The model under review builds one solid part; all positions refer to its coordinate system, in mm. A direction names the side the tool comes from. Coordinates: 2 decimals unless noted, no trailing zeros. Order: outer loops, then holes, each group sorted by start corner. A loop starts at its lowest first (then second) coordinate and runs counter-clockwise, first axis right, second up. Notation, with made-up numbers: M 31.5,57 L 83.5,57 A20 ccw 83.5,89 Z; hole C -28.75,-34.75 d1. An arc over 180 degrees is marked long. One line per item, written item: value.
```python
from build123d import *

# Parameters (mm, degrees)
SKETCH_2_R     = 5
SKETCH_2_R_2   = 3
CHAMFER_1_SIZE = 1


with BuildPart() as part:
    # По траектории1: sweep along a path in Эскиз1
    with BuildLine(Plane.XY) as sweep_1_path:
        Line((0, 0), (105, 0))
        ThreePointArc((105, 0), (123.47759065, -12.346331353), (119.142135624, -34.142135624))
        Line((119.142135624, -34.142135624), (95.857864376, -57.426406871))
        ThreePointArc((95.857864376, -57.426406871), (91.52240935, -63.914873848), (90, -71.568542495))
        Line((90, -71.568542495), (90, -100))
    # Эскиз2 → По траектории1 (sweep)
    with BuildSketch(Plane(origin=(0, 0, 0), x_dir=(0, 0, -1), z_dir=(1, 0, 0))):
        Circle(SKETCH_2_R)
        Circle(SKETCH_2_R_2, mode=Mode.SUBTRACT)
    sweep(path=sweep_1_path.line)

    # Фаска1
    chamfer_1_edges = [part.edges().sort_by_distance(p)[0] for p in [
        (90, -100, 5),
        (0, 0, 5),
    ]]
    chamfer(chamfer_1_edges, length=CHAMFER_1_SIZE)


solid = part.part
```
(1) For L1, parallel to Y at x = 81, z = 0; L2, parallel to X at y = -85.25, z = 0; L3, parallel to Y at x = 101, z = 1, list the stretches that pass through material, from the lowest coordinate up.
Geometry results:
L1: y = -5 to -3, 3 to 5
L2: x = 85 to 87, 93 to 95
L3: y = -59.21 to -56.28, -48.28 to -45.36, -4.9 to -2.83, 2.83 to 4.9
(2) We need section D-D, the plane y = -78. State the section outline as (x, z) points.
Geometry results:
outline: C 90,0 d10; hole C 90,0 d6
(3) We need section C-C, the plane x = 8. State the section outline as (y, z) points.
Geometry results:
outline: C 0,0 d10; hole C 0,0 d6
(4) Mouldability with a two-part tool opening along Y and no side actions: class faces 1 (the flat face through (93, -100, -1)), 2 (the cylindrical face through (85.12, -85.48, 1.08)), 3 (the cylindrical face through (103.886, -42.496, 1.084)) as +Y half, -Y half, draft (parallel to the pull), parting line (faces both ways), or undercut.
Geometry results:
face 1: -Y half
face 2: draft
face 3: undercut
(5) Tool access review of faces 4 (the flat face through (0, -3, 1)), 5 (the cylindrical face through (87.07, -85.98, 0.65)), 6 (the cylindrical face through (53.73, -4.88, 1.08)): name each direction out of +Z, -Z, +X, -X, +Y, -Y from which nothing blocks a thin tool from reaching the whole face with its end or side.
Geometry results:
face 4: +Z, -Z, -X, +Y, -Y
face 5: -Y
face 6: -X
(6) We need section A-A, the plane x = 90. Count the separate pieces of the cut face and the enclosed holes in it, plus the area to 3 significant figures.
Geometry results:
separate pieces: 2
enclosed holes: 1
area: 234 mm2
(7) Insertion check: pin 1 Ø2 at (x, z) = (82.5, -3) entering from -Y; pin 2 Ø2 at (x, z) = (102, -1) entering from -Y; pin 3 Ø5 at (y, z) = (0, 0) entering from +X. Each pin has a flat end and moves straight along its axis. Give the tip position at first contact, or say it passes through.
Geometry results:
pin 1: stops at y = -4.58
pin 2: stops at y = -59.24
pin 3: stops at x = 122.85
(8) We need section B-B, the plane z = 0. State the section outline as (x, y) points, plus the area to 3 significant figures.
Geometry results:
outline: M 0,-4 L 1,-5 L 105,-5 A15 cw 115.61,-30.61 L 92.32,-53.89 A25 ccw 85,-71.57 L 85,-99 L 86,-100 L 87,-100 L 87,-71.57 A23 cw 93.74,-55.31 L 117.02,-32.02 A17 ccw 105,-3 L 0,-3 Z; M 0,3 L 105,3 A23 cw 121.26,-36.26 L 97.98,-59.55 A17 ccw 93,-71.57 L 93,-100 L 94,-100 L 95,-99 L 95,-71.57 A15 cw 99.39,-60.96 L 122.68,-37.68 A25 ccw 105,5 L 1,5 L 0,4 Z
area: 915 mm2
